from build123d import *

# Parameters (mm, degrees)
SKETCH1_R                 = 17.9
BOSS_EXTRUDE1_DEPTH       = 21.8
FILLET1_R                 = 2.5
SKETCH2_R                 = 4.5
BOSS_EXTRUDE2_DEPTH       = 2.5
FILLET2_R                 = 0.5
M3X0_5_TAPPED_HOLE1_D     = 2.5
M3X0_5_TAPPED_HOLE1_DEPTH = 7.62
M3X0_5_TAPPED_HOLE1_TIP   = 0.751075774
SKETCH5_R                 = 1.5
BOSS_EXTRUDE3_DEPTH       = 12.5
SKETCH6_R                 = 6.35
BOSS_EXTRUDE4_DEPTH       = 2
BOSS_EXTRUDE5_START       = 1
SKETCH7_R                 = 1.5
BOSS_EXTRUDE5_DEPTH       = 1


with BuildPart() as part:
    # Sketch1 → Boss-Extrude1 (new body)
    with BuildSketch(Plane.XY):
        Circle(SKETCH1_R)
    extrude(amount=BOSS_EXTRUDE1_DEPTH)

    # Fillet1
    fillet1_edges = [part.edges().sort_by_distance(p)[0] for p in [
        (-17.9, 0, 21.8),
    ]]
    fillet(fillet1_edges, radius=FILLET1_R)

    # Sketch2 → Boss-Extrude2 (add)
    with BuildSketch(Plane.XY.offset(21.8)):
        Circle(SKETCH2_R)
    extrude(amount=BOSS_EXTRUDE2_DEPTH)

    # Fillet2
    fillet2_edges = [part.edges().sort_by_distance(p)[0] for p in [
        (-4.5, 0, 24.3),
    ]]
    fillet(fillet2_edges, radius=FILLET2_R)

    # M3x0.5 Tapped Hole1
    with Locations(Plane.XY.offset(21.8)):
        with Locations((0, 12.5), (0, -12.5), (12.5, 0), (-12.5, 0)):
            Hole(M3X0_5_TAPPED_HOLE1_D / 2, depth=M3X0_5_TAPPED_HOLE1_DEPTH)
            with Locations((0, 0, -(M3X0_5_TAPPED_HOLE1_DEPTH + M3X0_5_TAPPED_HOLE1_TIP / 2))):  # 118° drill point
                Cone(0, M3X0_5_TAPPED_HOLE1_D / 2, M3X0_5_TAPPED_HOLE1_TIP, mode=Mode.SUBTRACT)

    # Sketch5 → Boss-Extrude3 (add)
    with BuildSketch(Plane.XY.offset(24.3)):
        Circle(SKETCH5_R)
    extrude(amount=BOSS_EXTRUDE3_DEPTH)

    # Sketch6 → Boss-Extrude4 (add)
    with BuildSketch(Plane(origin=(0, 0, 0), x_dir=(-1, 0, 0), z_dir=(0, 0, -1))):
        Circle(SKETCH6_R)
    extrude(amount=BOSS_EXTRUDE4_DEPTH)

    # Sketch7 → Boss-Extrude5 (add)
    with BuildSketch(Plane(origin=(0, 0, -2), x_dir=(-1, 0, 0), z_dir=(0, 0, -1)).offset(BOSS_EXTRUDE5_START)):
        with Locations(Location((0, 0, 0), (0, 0, 180))):
            Circle(SKETCH7_R)
    extrude(amount=-BOSS_EXTRUDE5_DEPTH)


solid = part.part
Build history of the part. All positions in model axes, mm. A direction names the side the tool comes from. Round coordinates to 2 decimals unless told otherwise and drop trailing zeros. Write each loop counter-clockwise with the first axis right and the second up, starting at its lowest first coordinate (ties: lowest second). Pieces come first, ordered by that corner, then holes. Notation, with made-up numbers: (80, 20) - (114, 20) arc R15 cw to (114, 27) - close; hole circle Ø4 at (76, 30.5). An arc over 180 degrees is marked (long way). One line per question, with ' | ' between items.
1. Drill centre lines: line 1 along Y through (x, z) = (0, 19.5); line 2 along Z through (x, y) = (-4, -12.5); line 3 along Y through (x, z) = (12, 16). Where is each one in solid material? Low to high. Write a range as from..to.
Results are:
line 1: -17.89..-13.75, -11.25..11.25, 13.75..17.89 | line 2: 0..21.8 | line 3: -13.28..-1.15, 1.15..13.28
2. Mould opens along X. For faces 1 (the face through (0, 0, 36.8)), 2 (the face through (-14.2, -10.9, 9.5)), 3 (the face through (13.75, 0.05, 17.94)) say: released by +X, released by -X, zero draft, split by the parting line, or undercut.
Results are:
face 1: zero draft | face 2: split by the parting line | face 3: undercut
3. Band-saw the part on B-B, the plane z = 29.5. Write the cut outline in (x, y), and give its area (3 significant figures).
Results are:
outline: circle Ø3 at (0, 0) | area: 7.07 mm^2
4. Drop flat-ended pins along their axis: pin 1 Ø8 at (y, z) = (-9, 2) entering from +X; pin 2 Ø5 at (y, z) = (10, 14.5) entering from -X; pin 3 Ø10 at (x, y) = (3, 3) entering from -Z; pin 4 Ø8 at (x, z) = (-3, 11) entering from +Y. Give the stop position or say it passes through.
Results are:
pin 1: x = 17.19 | pin 2: x = -16.25 | pin 3: z = -3 | pin 4: y = 17.9
5. Band-saw the part on A-A, the plane z = 12.5. Write the cut outline in (x, y).
Results are:
outline: circle Ø35.8 at (0, 0)
6. Tool access for faces 4 (the face through (0.16, -11.26, 17.94)), 5 (the face through (0, 0, -3)), 6 (the face through (8, 0, 0)): list every direction of +Z, -Z, +X, -X, +Y, -Y with a clear straight run to the whole face (end or side of a thin tool).
Results are:
face 4: +Z | face 5: -Z, +X, -X, +Y, -Y | face 6: -Z
